Build history of the part. All positions in model axes, mm. Give positions to 0.01 mm unless a question says otherwise; leave off trailing zeros. Order: outer loops, then holes, each group sorted by start corner. A loop starts at its lowest first (then second) coordinate and runs counter-clockwise, first axis right, second up. Notation, with made-up numbers: (4, 84.5) - (8, 84.5) arc R27 ccw to (8, 113.5) - close; hole circle Ø10 at (73.5, 26). An arc over 180 degrees is marked (long way). Use a Markdown table: item, result. Add a question column.
(1) Slice it at D-D (x = -0.75). Write the cut outline in (y, z).
(2) Flat gauge pins, fed straight in: pin 1 (1.5 mm diameter, centred on y = -1, z = 1, fed in from -X); pin 2 (2 mm diameter, centred on x = -0.5, z = 2, fed in from +Y). Where does each tip first touch, or does it go through?
(3) Mould opens along Z. For faces 1 (the face through (-1.1, 0.4, 0)), 2 (the face through (-1, 0, -2)), 3 (the face through (0, -1, 2)) say: +Z half, -Z half, draft (parallel to the pull), parting line (faces both ways), or undercut.
(4) Wall check: line 1 (Z direction, x = -0.2, y = 0); line 2 (Y direction, x = -0.85, z = -1.5); line 3 (Z direction, x = -1.1, y = 1.5). Give the ranges that are in metal, low to high.
(5) Slice it at C-C (z = -1.5). Write the cut outline in (x, y), then the cut area to 3 significant figures.
(6) Slice it at B-B (x = 0). Write the cut outline in (y, z), then the cut area to 3 significant figures.
(7) Slice it at A-A (y = 0). Write the cut outline in (x, z).
from build123d import *

# Parameters (mm, degrees)
F0_R           = 1
F1_DEPTH       = 4
F2_R           = 2
F3_DEPTH       = 3
F6_D           = 1
F6_CSINK_D     = 2.9
F6_CSINK_ANGLE = 90
F7_W           = 3.740538
F7_H           = 4.958128
F8_DEPTH       = 25
F8_DEPTH_BACK  = 25


with BuildPart() as f1:
    # F0 (on Top) → F1 (new body)
    with BuildSketch(Plane.XY):
        Circle(F0_R)
    extrude(amount=F1_DEPTH)

    # F2 (on face) → F3 (join)
    with BuildSketch(Plane(origin=(0, 0, 0), x_dir=(1, 0, 0), z_dir=(0, 0, -1))):
        Circle(F2_R)
    extrude(amount=F3_DEPTH)

    # F6 (through all)
    with Locations(Plane.YZ.offset(1.5)):
        with Locations((0, -1.5)):
            CounterSinkHole(F6_D / 2, F6_CSINK_D / 2, counter_sink_angle=F6_CSINK_ANGLE)

    # F7 (on Front) → F8 (cut, two sides)
    with BuildSketch(Plane.XZ) as f8_sk:
        with Locations((3.370269, -2.379064)):
            Rectangle(F7_W, F7_H)
    extrude(amount=F8_DEPTH, mode=Mode.SUBTRACT)
    extrude(f8_sk.sketch, amount=-F8_DEPTH_BACK, mode=Mode.SUBTRACT)


solid = f1.part
Solution:
| question | item | result |
|---|---|---|
| 1 | outline | (-1.85, -3) - (1.85, -3) - (1.85, 0) - (0.66, 0) - (0.66, 4) - (-0.66, 4) - (-0.66, 0) - (-1.85, 0) - close; hole circle Ø1 at (0, -1.5) |
| 2 | pin 1 | x = -0.97 |
| 2 | pin 2 | y = 1 |
| 3 | face 1 | +Z half |
| 3 | face 2 | undercut |
| 3 | face 3 | draft |
| 4 | line 1 | -3 to -2, -1 to 4 |
| 4 | line 2 | -1.81 to -0.5, 0.5 to 1.81 |
| 4 | line 3 | -3 to 0 |
| 5 | outline | (-1.94, -0.5) arc R2 ccw to (1.44, -1.39) - (0.55, -0.5) - close; (-1.94, 0.5) - (0.55, 0.5) - (1.44, 1.39) arc R2 ccw to start |
| 5 | area | 7.29 mm2 |
| 6 | outline | (-2, -3) - (2, -3) - (2, 0) - (1, 0) - (1, 4) - (-1, 4) - (-1, 0) - (-2, 0) - close; hole circle Ø1 at (0, -1.5) |
| 6 | area | 19.2 mm2 |
| 7 | outline | (-2, -3) - (1.5, -3) - (1.5, -2.95) - (0.55, -2) - (-2, -2) - close; (-2, -1) - (0.55, -1) - (1.5, -0.05) - (1.5, 0) - (1, 0) - (1, 4) - (-1, 4) - (-1, 0) - (-2, 0) - close |
